Design review of the part built by this model. Coordinates are the model's own, in mm. Face numbers are marked on the shaded views. A direction names the side the tool comes from. Coordinates: 2 decimals unless noted, no trailing zeros. Write each loop counter-clockwise with the first axis right and the second up, starting at its lowest first coordinate (ties: lowest second). Pieces come first, ordered by that corner, then holes. Notation, with made-up numbers: (0, -3.5) -> (27, -3.5) arc R11 ccw to (27, 17.5) -> close; hole circle Ø1 at (-26.5, -3). An arc over 180 degrees is marked (long way). Write item = value, one per line. Start each with the question number.
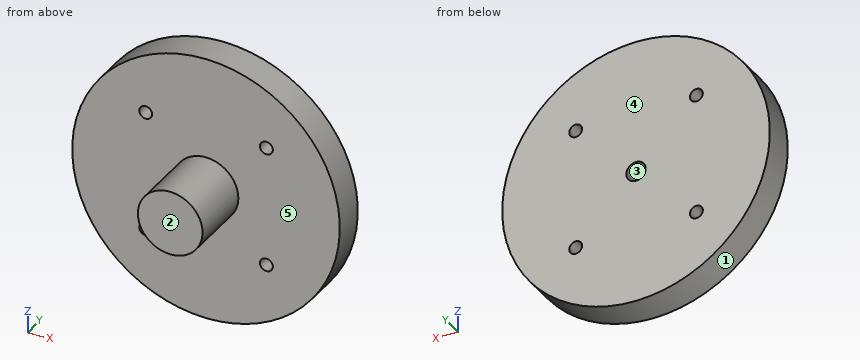
```python
from build123d import *

# Parameters (mm, degrees)
SKETCH1_R               = 12.419595949
SKETCH1_R_2             = 0.9
SKETCH1_R_3             = 0.6
DISCO_APONEUROSIS_DEPTH = 3


with BuildPart() as part:
    # Sketch1 → Disco_aponeurosis (new body)
    with BuildSketch(Plane(origin=(0, -209, 0), x_dir=(1, 0, 0), z_dir=(0, 1, 0))):
        with Locations(Location((0, 0, 0), (0, 0, 270))):
            Circle(SKETCH1_R)
        with Locations(Location((0, 0, 0), (0, 0, 270))):
            Circle(SKETCH1_R_2, mode=Mode.SUBTRACT)
        with Locations(Location((5.6, 5.6, 0), (0, 0, 270))):
            Circle(SKETCH1_R_3, mode=Mode.SUBTRACT)
        with Locations(Location((-5.6, 5.6, 0), (0, 0, 270))):
            Circle(SKETCH1_R_3, mode=Mode.SUBTRACT)
        with Locations(Location((-5.6, -5.6, 0), (0, 0, 270))):
            Circle(SKETCH1_R_3, mode=Mode.SUBTRACT)
        with Locations(Location((5.6, -5.6, 0), (0, 0, 270))):
            Circle(SKETCH1_R_3, mode=Mode.SUBTRACT)
    extrude(amount=DISCO_APONEUROSIS_DEPTH)

    # Sketch2 → Boca_tendon (revolve)
    with BuildSketch(Plane.XY, mode=Mode.PRIVATE) as boca_tendon_sk:
        Polygon((0, -209), (3, -209), (3, -215), (1.2, -215), (0, -215), align=None)
    revolve(boca_tendon_sk.sketch.rotate(Axis((0, -219, 0), (0, 1, 0)), 90), axis=Axis((0, -219, 0), (0, 1, 0)))


solid = part.part
```
(1) Mouldability with a two-part tool opening along Z and no side actions: class the marked faces 1, 2 and 3 as pulls with the +Z half, pulls with the -Z half, needs draft (parallel to the pull), parting line crosses it, or undercut.
(2) Take a section at A-A, the plane z = 0. State the section outline as (x, y) points, then the cut area to 3 significant figures.
(3) Take a section at C-C, the plane x = -5.6. State the section outline as (y, z) points.
(4) For pin 1 Ø1.6 at (x, z) = (-5.6, -5.6) entering from -Y; pin 2 Ø0.7 at (x, z) = (5.6, -5.6) entering from -Y; pin 3 Ø3 at (x, z) = (2.5, 2.5) entering from -Y; pin 4 Ø0.5 at (x, z) = (0, 0.5) entering from +Y, all flat-tipped, find the tip position at first contact; note any pin that passes through.
(5) Take a section at D-D, the plane z = -5.6. State the section outline as (x, y) points.
(6) For line 1 (X direction, y = -208.3, z = -5.6); line 2 (Y direction, x = 10, z = -1); line 3 (X direction, y = -208, z = -1.5), list the stretches that pass through material, from the lowest coordinate up.
(7) Take a section at B-B, the plane y = -207.25. State the section outline as (x, z) points.
(8) For the marked faces 4 and 5, list the 3-axis set-ups (+Z, -Z, +X, -X, +Y, -Y) from which the entire face can be reached by the end or side of a thin tool; tool diameter is ignored.
Report:
q1.face_1 = parting line crosses it
q1.face_2 = needs draft
q1.face_3 = undercut
q2.outline = (-12.42, -209) -> (-3, -209) -> (-3, -215) -> (3, -215) -> (3, -209) -> (12.42, -209) -> (12.42, -206) -> (0.9, -206) -> (0.9, -209) -> (-0.9, -209) -> (-0.9, -206) -> (-12.42, -206) -> close
q2.area = 105 mm2
q3.outline = (-209, -11.09) -> (-206, -11.09) -> (-206, -6.2) -> (-209, -6.2) -> close; (-209, -5) -> (-206, -5) -> (-206, 5) -> (-209, 5) -> close; (-209, 6.2) -> (-206, 6.2) -> (-206, 11.09) -> (-209, 11.09) -> close
q4.pin_1 = -209
q4.pin_2 = through
q4.pin_3 = -215
q4.pin_4 = -209
q5.outline = (-11.09, -209) -> (-6.2, -209) -> (-6.2, -206) -> (-11.09, -206) -> close; (-5, -209) -> (5, -209) -> (5, -206) -> (-5, -206) -> close; (6.2, -209) -> (11.09, -209) -> (11.09, -206) -> (6.2, -206) -> close
q6.line_1 = -11.09 to -6.2, -5 to 5, 6.2 to 11.09
q6.line_2 = -209 to -206
q6.line_3 = -12.33 to 12.33
q7.outline = circle Ø24.84 at (0, 0); hole circle Ø1.2 at (-5.6, -5.6); hole circle Ø1.2 at (-5.6, 5.6); hole circle Ø1.8 at (0, 0); hole circle Ø1.2 at (5.6, -5.6); hole circle Ø1.2 at (5.6, 5.6)
q8.face_4 = +Z, -Z, +X, -X, +Y
q8.face_5 = -Y
